Work out the finished part from the listing and answer in its coordinate system (mm). A direction names the side the tool comes from. Round coordinates to 2 decimals unless told otherwise and drop trailing zeros. Write each loop counter-clockwise with the first axis right and the second up, starting at its lowest first coordinate (ties: lowest second). Pieces come first, ordered by that corner, then holes. Notation, with made-up numbers: (71.5, 14) - (112.5, 14) arc R12 cw to (112.5, 31) - close; hole circle Ø4 at (39.25, 32.25). An arc over 180 degrees is marked (long way). Answer as a JSON object with one key per item and string values.
```python
from build123d import *

# Parameters (mm, degrees)
BOSS_EXTRUDE1_DEPTH = 2.2
SKETCH2_R           = 7.5
BOSS_EXTRUDE2_DEPTH = 14
SKETCH4_R           = 2
BOSS_EXTRUDE3_DEPTH = 117
SKETCH6_R           = 17.4
BOSS_EXTRUDE4_DEPTH = 1.5
SKETCH7_R           = 1.5
CUT_EXTRUDE1_DEPTH  = 1


with BuildPart() as part:
    # Sketch1 → Boss-Extrude1 (new body)
    with BuildSketch(Plane.XY):
        with BuildLine():
            Line((-3.35, 16.35), (-3.35, 10.103341032))
            ThreePointArc((-3.35, 10.103341032), (-3.514699292, 9.553547682), (-3.954545455, 9.184855483))
            ThreePointArc((-3.954545455, 9.184855483), (-7.071067812, 7.071067812), (-9.184855483, 3.954545455))
            ThreePointArc((-9.184855483, 3.954545455), (-9.553547682, 3.514699292), (-10.103341032, 3.35))
            Line((-10.103341032, 3.35), (-16.35, 3.35))
            ThreePointArc((-16.35, 3.35), (-19.7, 0), (-16.35, -3.35))
            Line((-16.35, -3.35), (-10.103341032, -3.35))
            ThreePointArc((-10.103341032, -3.35), (-9.553547682, -3.514699292), (-9.184855483, -3.954545455))
            ThreePointArc((-9.184855483, -3.954545455), (-7.071067812, -7.071067812), (-3.954545455, -9.184855483))
            ThreePointArc((-3.954545455, -9.184855483), (-3.514699292, -9.553547682), (-3.35, -10.103341032))
            Line((-3.35, -10.103341032), (-3.35, -16.35))
            ThreePointArc((-3.35, -16.35), (0, -19.7), (3.35, -16.35))
            Line((3.35, -16.35), (3.35, -10.103341032))
            ThreePointArc((3.35, -10.103341032), (3.514699292, -9.553547682), (3.954545455, -9.184855483))
            ThreePointArc((3.954545455, -9.184855483), (7.071067812, -7.071067812), (9.184855483, -3.954545455))
            ThreePointArc((9.184855483, -3.954545455), (9.553547682, -3.514699292), (10.103341032, -3.35))
            Line((10.103341032, -3.35), (16.35, -3.35))
            ThreePointArc((16.35, -3.35), (19.7, 0), (16.35, 3.35))
            Line((16.35, 3.35), (10.103341032, 3.35))
            ThreePointArc((10.103341032, 3.35), (9.553547682, 3.514699292), (9.184855483, 3.954545455))
            ThreePointArc((9.184855483, 3.954545455), (7.071067812, 7.071067812), (3.954545455, 9.184855483))
            ThreePointArc((3.954545455, 9.184855483), (3.514699292, 9.553547682), (3.35, 10.103341032))
            Line((3.35, 10.103341032), (3.35, 16.35))
            ThreePointArc((3.35, 16.35), (0, 19.7), (-3.35, 16.35))
        make_face()
        with BuildLine():
            Line((16.5, 1.5), (9.2, 1.5))
            ThreePointArc((9.2, 1.5), (7.7, 0), (9.2, -1.5))
            Line((9.2, -1.5), (16.5, -1.5))
            ThreePointArc((16.5, -1.5), (18, 0), (16.5, 1.5))
        make_face(mode=Mode.SUBTRACT)
        with BuildLine():
            Line((-1.5, -9.2), (-1.5, -16.5))
            ThreePointArc((-1.5, -16.5), (0, -18), (1.5, -16.5))
            Line((1.5, -16.5), (1.5, -9.2))
            ThreePointArc((1.5, -9.2), (0, -7.7), (-1.5, -9.2))
        make_face(mode=Mode.SUBTRACT)
        with BuildLine():
            Line((-9.2, 1.5), (-16.5, 1.5))
            ThreePointArc((-16.5, 1.5), (-18, 0), (-16.5, -1.5))
            Line((-16.5, -1.5), (-9.2, -1.5))
            ThreePointArc((-9.2, -1.5), (-7.7, 0), (-9.2, 1.5))
        make_face(mode=Mode.SUBTRACT)
        with BuildLine():
            Line((1.5, 9.2), (1.5, 16.5))
            ThreePointArc((1.5, 16.5), (0, 18), (-1.5, 16.5))
            Line((-1.5, 16.5), (-1.5, 9.2))
            ThreePointArc((-1.5, 9.2), (0, 7.7), (1.5, 9.2))
        make_face(mode=Mode.SUBTRACT)
    extrude(amount=BOSS_EXTRUDE1_DEPTH)

    # Sketch2 → Boss-Extrude2 (add)
    with BuildSketch(Plane.XY.offset(2.2)):
        Circle(SKETCH2_R)
    extrude(amount=BOSS_EXTRUDE2_DEPTH)

    # Sketch3 → Revolve1 (revolve)
    with BuildSketch(Plane(origin=(0, 0, 0), x_dir=(1, 0, 0), z_dir=(0, 1, 0)), mode=Mode.PRIVATE) as revolve1_sk:
        Polygon((0, -16.2), (7.5, -16.2), (4.5, -29.2), (0, -29.2), align=None)
    revolve(revolve1_sk.sketch.rotate(Axis((0, 0, 16.2), (0, 0, 1)), 180), axis=Axis((0, 0, 16.2), (0, 0, 1)))

    # Sketch4 → Boss-Extrude3 (add)
    with BuildSketch(Plane.XY.offset(29.2)):
        Circle(SKETCH4_R)
    extrude(amount=BOSS_EXTRUDE3_DEPTH)

    # Sketch5 → Revolve2 (revolve)
    with BuildSketch(Plane(origin=(0, 0, 0), x_dir=(1, 0, 0), z_dir=(0, 1, 0)), mode=Mode.PRIVATE) as revolve2_sk:
        Polygon((0, -146.2), (3.4, -146.2), (7, -153.7), (0, -153.7), align=None)
    revolve(revolve2_sk.sketch.rotate(Axis((0, 0, 146.2), (0, 0, 1)), 180), axis=Axis((0, 0, 146.2), (0, 0, 1)))

    # Sketch6 → Boss-Extrude4 (add)
    with BuildSketch(Plane.XY.offset(153.7)):
        Circle(SKETCH6_R)
    extrude(amount=BOSS_EXTRUDE4_DEPTH)

    # Sketch7 → Cut-Extrude1 (cut)
    with BuildSketch(Plane.XY.offset(155.2)):
        Circle(SKETCH7_R)
    extrude(amount=-CUT_EXTRUDE1_DEPTH, mode=Mode.SUBTRACT)


solid = part.part
```
Item 1: Consider line 1 along Y through (x, z) = (0, 154.65); line 2 along Z through (x, y) = (14, -2.5); line 3 along Z through (x, y) = (-8, 14.5). Determine where each line is inside the solid, lowest interval first.
Results found:
{"line 1": "-17.4 to -1.5, 1.5 to 17.4", "line 2": "0 to 2.2, 153.7 to 155.2", "line 3": "153.7 to 155.2"}
Item 2: A cutting plane is placed at B-B (z = 37). Write down the section's boundary in (x, y), and give its area (3 significant figures).
Results found:
{"outline": "circle Ø4 at (0, 0)", "area": "12.6 mm²"}
Item 3: For faces 5 (the cylindrical face through (-0.1, -19.7, 1.1)), 6 (the cylindrical face through (-19.7, 0.1, 1.1)), 7 (the cylindrical face through (-7.11, -7.03, 1.08)), 8 (the cylindrical face through (19.7, -0.1, 1.1)), 9 (the cylindrical face through (-7.493, 0.33, 9.102)), determine the directions among +Z, -Z, +X, -X, +Y, -Y from which every point of the face is accessible in a straight line to the end or side of a thin tool.
Results found:
{"face 5": "-Z, -Y", "face 6": "-Z, -X", "face 7": "-Z, -X, -Y", "face 8": "-Z, +X", "face 9": "none"}
Item 4: Each of these flat-tipped pins is pushed along its axis until it touches: P1, Ø1.8, axis at x = -12, z = 0.5, coming from the -Y side; P2, Ø1.1, axis at y = 11.5, z = 1.5, coming from the +X side; P3, Ø4, axis at x = 0, y = 0, coming from the +Z side; P4, Ø1.1, axis at x = 14, z = 0.5, coming from the +Y side. Where does it stop, or does it pass through?
Results found:
{"P1": "y = -3.35", "P2": "x = 3.35", "P3": "z = 155.2", "P4": "y = 3.35"}
Item 5: Determine the mould class of faces 1 (the cylindrical face through (7.03, -7.11, 1.08)), 2 (the cylindrical face through (-1.5, 0.07, 154.71)), 3 (the flat face through (-0.2, -7.5, 153.7)), 4 (the flat face through (0, 0, 154.2)) for opening direction X: pulls with the +X half, pulls with the -X half, needs draft (parallel to the pull), parting line crosses it, or undercut.
Results found:
{"face 1": "pulls with the +X half", "face 2": "undercut", "face 3": "needs draft", "face 4": "undercut"}
Item 6: A cutting plane is placed at A-A (y = 15). Write down the section's boundary in (x, z), and give its area (3 significant figures).
Results found:
{"outline": "(-8.82, 153.7) - (8.82, 153.7) - (8.82, 155.2) - (-8.82, 155.2) - close; (-3.35, 0) - (-1.5, 0) - (-1.5, 2.2) - (-3.35, 2.2) - close; (1.5, 0) - (3.35, 0) - (3.35, 2.2) - (1.5, 2.2) - close", "area": "34.6 mm²"}
